Can you work these out from the model? Positions are in its coordinate system, mm. A direction names the side the tool comes from. Round coordinates to 2 decimals unless told otherwise and drop trailing zeros. Order: outer loops, then holes, each group sorted by start corner. A loop starts at its lowest first (then second) coordinate and runs counter-clockwise, first axis right, second up. Notation, with made-up numbers: (34, 58.5) -> (72, 58.5) arc R18 ccw to (72, 81.5) -> close; hole circle Ø6 at (-34.75, 66). An arc over 180 degrees is marked (long way). Use a Markdown table: item, result. Add a question column.
Q1. If we section it at A-A on x = 7: List the corners of the cut face in (y, z) for me.
Q2. I'm going to push flat-ended pins straight in: pin 1 Ø1.5 at (y, z) = (2, -120) entering from +X; pin 2 Ø2 at (y, z) = (5, -62) entering from +X; pin 3 Ø0.9 at (y, z) = (1.5, 185) entering from +X; pin 4 Ø0.9 at (x, y) = (155.5, 1) entering from +Z. Where does each tip first touch, or does it pass through?
Q3. I need wall thicknesses on line 1 along X through (y, z) = (2.65, 4.5); line 2 along Y through (x, z) = (-76.5, 105.5); line 3 along X through (y, z) = (2.1, 41.5). Which ranges of each line are inside material? Lowest first, please. Write a range as [from, to].
Q4. We'd pull the mould along Z, two halves only. Please class faces 3 (the face through (-93.37, 4.48, 156.32)), 4 (the face through (117, 6, 146)): +Z half, -Z half, draft (parallel to the pull), parting line (faces both ways), or undercut.
Q5. If we section it at D-D on z = 143.5: List the corners of the cut face in (x, y) for me, plus the area to 3 significant figures.
Q6. If we section it at C-C on y = 5: List the corners of the cut face in (x, z) for me.
Q7. If we section it at B-B on z = 45: List the corners of the cut face in (x, y) for me.
Q8. For faces 1 (the face through (-94, 6, -82)), 2 (the face through (125.62, 4.48, -87.05)), which set-ups out of +Z, -Z, +X, -X, +Y, -Y let a thin tool reach every point of the face, with its end or its side?
```python
from build123d import *

# Parameters (mm, degrees)
EXTRUDE_1_DEPTH = 3
SKETCH_2_R      = 10
EXTRUDE_3_DEPTH = 6


with BuildPart() as part:
    # Эскиз1 → Бобышка-Вытянуть1 (new body)
    with BuildSketch(Plane(origin=(0, 0, 0), x_dir=(1, 0, 0), z_dir=(0, 1, 0))):
        Polygon((-130.811243507, 121.669438521), (-84.811243507, 121.669438521), (-84.811243507, 118.669438521), (-36.311243507, 118.669438521), (-36.311243507, 121.669438521), (12.188756493, 121.669438521), (12.188756493, 118.669438521), (60.688756493, 118.669438521), (60.688756493, 121.669438521), (109.188756493, 121.669438521), (109.188756493, 118.669438521), (157.188756493, 118.669438521), (157.188756493, 70.169438521), (154.188756493, 70.169438521), (154.188756493, 18.869438521), (157.188756493, 18.869438521), (157.188756493, -33.830561479), (154.188756493, -33.830561479), (154.188756493, -83.730561479), (157.188756493, -83.730561479), (157.188756493, -135.030561479), (154.188756493, -135.030561479), (154.188756493, -183.330561479), (108.688756493, -183.330561479), (108.688756493, -186.330561479), (60.188756493, -186.330561479), (60.188756493, -183.330561479), (11.688756493, -183.330561479), (11.688756493, -186.330561479), (-36.811243507, -186.330561479), (-36.811243507, -183.330561479), (-85.311243507, -183.330561479), (-85.311243507, -186.330561479), (-133.811243507, -186.330561479), (-133.811243507, -135.030561479), (-130.811243507, -135.030561479), (-130.811243507, -83.730561479), (-133.811243507, -83.730561479), (-133.811243507, -32.430561479), (-130.811243507, -32.430561479), (-130.811243507, 18.869438521), (-133.811243507, 18.869438521), (-133.811243507, 70.169438521), (-130.811243507, 70.169438521), align=None)
    extrude(amount=EXTRUDE_1_DEPTH)

    # Эскиз2 → Бобышка-Вытянуть3 (add)
    with BuildSketch(Plane.XZ):
        with Locations(Location((-93.811243507, 146.330561479, 0), (0, 0, 270))):
            Circle(SKETCH_2_R)
        with Locations(Location((117.188756493, 146.330561479, 0), (0, 0, 270))):
            Circle(SKETCH_2_R)
        with Locations(Location((117.188756493, -81.669438521, 0), (0, 0, 270))):
            Circle(SKETCH_2_R)
        with Locations(Location((-93.811243507, -81.669438521, 0), (0, 0, 270))):
            Circle(SKETCH_2_R)
    extrude(amount=-EXTRUDE_3_DEPTH)


solid = part.part
```
Answer below:
| question | item | result |
|---|---|---|
| 1 | outline | (0, -121.67) -> (3, -121.67) -> (3, 186.33) -> (0, 186.33) -> close |
| 2 | pin 1 | x = 109.19 |
| 2 | pin 2 | through |
| 2 | pin 3 | x = 108.69 |
| 2 | pin 4 | z = 135.03 |
| 3 | line 1 | [-130.81, 157.19] |
| 3 | line 2 | [0, 3] |
| 3 | line 3 | [-133.81, 154.19] |
| 4 | face 3 | undercut |
| 4 | face 4 | draft |
| 5 | outline | (-133.81, 0) -> (154.19, 0) -> (154.19, 3) -> (126.78, 3) -> (126.78, 6) -> (107.6, 6) -> (107.6, 3) -> (-84.22, 3) -> (-84.22, 6) -> (-103.4, 6) -> (-103.4, 3) -> (-133.81, 3) -> close |
| 5 | area | 979 mm² |
| 6 | outline | circle Ø20 at (-93.81, -81.67); circle Ø20 at (-93.81, 146.33); circle Ø20 at (117.19, -81.67); circle Ø20 at (117.19, 146.33) |
| 7 | outline | (-133.81, 0) -> (154.19, 0) -> (154.19, 3) -> (-133.81, 3) -> close |
| 8 | face 1 | +Z, -Z, +X, -X, +Y |
| 8 | face 2 | +Y |
